from build123d import *

# Parameters (mm, degrees)
CROQUIS1_W              = 15
CROQUIS1_H              = 5
SALIENTE_EXTRUIR1_DEPTH = 1050


with BuildPart() as part:
    # Croquis1 → Saliente-Extruir1 (new body)
    with BuildSketch(Plane.XY):
        Polygon((-5, 0), (0, 0), (0, 34), (-5, 34), (-5, 29), align=None)
        with Locations((-12.5, 31.5)):
            Rectangle(CROQUIS1_W, CROQUIS1_H)
    extrude(amount=-SALIENTE_EXTRUIR1_DEPTH)


solid = part.part
Model file for the job. Use its own axes, mm. A direction names the side the tool comes from. Give positions to 0.01 mm unless a question says otherwise; leave off trailing zeros. Write each loop counter-clockwise with the first axis right and the second up, starting at its lowest first coordinate (ties: lowest second). Pieces come first, ordered by that corner, then holes. Notation, with made-up numbers: M 71,-12 L 77,-12 A19 cw 77,-5 Z; hole C -31,34.25 d2. An arc over 180 degrees is marked long. One line per item, written item: value. Start each with the question number.
Q1. Drop flat-ended pins along their axis: pin 1 Ø10 at (x, y) = (-6.5, 18) entering from -Z; pin 2 Ø8.5 at (y, z) = (18, -733) entering from -X; pin 3 Ø12 at (x, z) = (-14, -431.5) entering from -Y; pin 4 Ø1.5 at (x, y) = (-6.5, 10) entering from +Z. Give the stop position or say it passes through.
Q2. Saw through at C-C, the plane x = -16. Write the cut outline in (y, z).
Q3. Probe probe 1 along Y at (x, z) = (-12, -53); probe 2 along X at (y, z) = (14.5, -158). List the from-to ranges inside material, lowest first. Write a range as [from, to].
Q4. Saw through at A-A, the plane z = -225.5. Write the cut outline in (x, y).
Q5. Saw through at B-B, the plane y = 16. Write the cut outline in (x, z).
Q6. 3-axis set-ups, long thin cutter, end or side, ignore diameter. For faces 1 (the flat face through (-4, 21, -1050)), 2 (the flat face through (-5, 15, -518)): which of +Z, -Z, +X, -X, +Y, -Y reach the whole face in a straight line?
Output values:
1. pin 1: stops at z = -1050
1. pin 2: stops at x = -5
1. pin 3: stops at y = 29
1. pin 4: passes through
2. outline: M 29,-1050 L 34,-1050 L 34,0 L 29,0 Z
3. probe 1: y = [29, 34]
3. probe 2: x = [-5, 0]
4. outline: M -20,29 L -5,29 L -5,0 L 0,0 L 0,34 L -20,34 Z
5. outline: M -5,-1050 L 0,-1050 L 0,0 L -5,0 Z
6. face 1: -Z, +X, -X, +Y, -Y
6. face 2: +Z, -Z, -X, -Y
